Source: CAD feature listing. Evaluate the final solid. Frame: model axes, mm. Coordinates: 2 decimals unless noted, no trailing zeros. Order: outer loops, then holes, each group sorted by start corner. A loop starts at its lowest first (then second) coordinate and runs counter-clockwise, first axis right, second up.
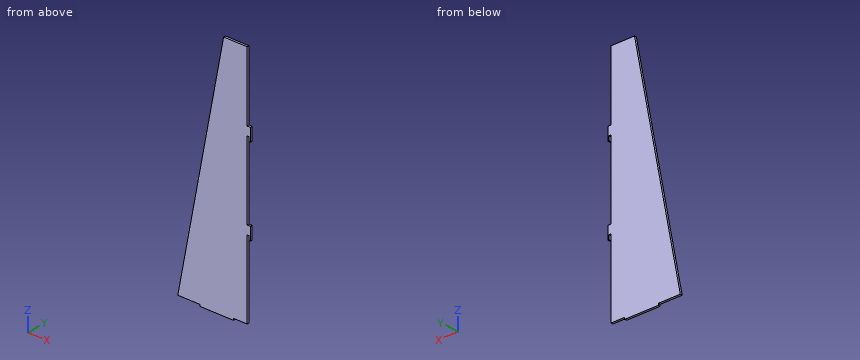
```python
from build123d import *

# Parameters (mm, degrees)
F1_DEPTH = 2.5
F3_DEPTH = 25


with BuildPart() as f1:
    # F0 (on Front) → F1 (new body)
    with BuildSketch(Plane.XZ):
        Polygon((-31.706513, 280), (-86.133, 0), (-60, 0), (-60, -2), (-20, -2), (-20, 0), (0, 0), (0, 280), align=None)
    extrude(amount=F1_DEPTH)

    # F2 (on Front) → F3 (cut)
    with BuildSketch(Plane.XZ):
        Polygon((25.523714, 0), (25.523714, 285.471179), (-3.88, 285.471179), (-3.88, 200), (3.67, 200), (3.67, 185), (-1.33, 185), (-1.33, 190), (-3.88, 190), (-3.88, 100), (3.67, 100), (3.67, 85), (-1.33, 85), (-1.33, 90), (-3.88, 90), (-3.88, 0), align=None)
    extrude(amount=F3_DEPTH, mode=Mode.SUBTRACT)


solid = f1.part
```
1. Ray query, line 1 (Z direction, x = -15.5, y = -1.25); line 2 (X direction, y = -1.35, z = 178); line 3 (X direction, y = -0.65, z = 262.5). Return the intervals inside material, ascending.
Findings:
line 1: z = 0 to 280
line 2: x = -51.53 to -3.88
line 3: x = -35.11 to -3.88
2. Section query B-B on z = 180.5. Return loops of the section in (x, y).
Findings:
outline: (-51.05, -2.5) - (-3.88, -2.5) - (-3.88, 0) - (-51.05, 0) - close
3. Section query A-A on y = -1.95. Return loops of the section in (x, z), plus the area to 3 significant figures.
Findings:
outline: (-86.13, 0) - (-60, 0) - (-60, -2) - (-20, -2) - (-20, 0) - (-3.88, 0) - (-3.88, 90) - (-1.33, 90) - (-1.33, 85) - (0, 85) - (0, 100) - (-3.88, 100) - (-3.88, 190) - (-1.33, 190) - (-1.33, 185) - (0, 185) - (0, 200) - (-3.88, 200) - (-3.88, 280) - (-31.71, 280) - close
area: 15,600 mm2
4. Pin query (flat end, axial travel): P1, Ø1, axis at y = -2, z = -1.5, coming from the -X side; P2, Ø1.2, axis at y = -1.5, z = 148.5, coming from the +X side; P3, Ø1.2, axis at x = -15.5, y = -1, coming from the -Z side. Return the tip coordinate at first contact, or that it passes through.
Findings:
P1: stops at x = -60
P2: stops at x = -3.88
P3: stops at z = 0
5. Section query C-C on x = -70. Return loops of the section in (y, z).
Findings:
outline: (-2.5, 0) - (0, 0) - (0, 83) - (-2.5, 83) - close
